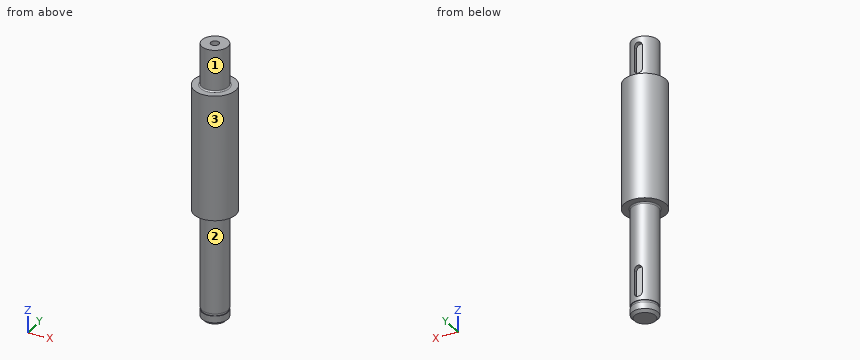
```python
from build123d import *

# Parameters (mm, degrees)
SKETCH1_R                          = 12.7
BOSS_EXTRUDE1_DEPTH                = 38.1
SKETCH3_R                          = 7.9375
BOSS_EXTRUDE2_DEPTH                = 66.675
SKETCH8_R                          = 12.7
SKETCH8_R_2                        = 7.4676
CUT_EXTRUDE1_DEPTH                 = 0.7112
BOSS_EXTRUDE3_START                = 25.4
SKETCH9_R                          = 7.9375
BOSS_EXTRUDE3_DEPTH                = 25.4
FILLET1_R                          = 0.79375
F_1_4_20_TAPPED_HOLE1_D            = 5.1054
F_1_4_20_TAPPED_HOLE1_DEPTH        = 38.1
F_1_4_20_TAPPED_HOLE1_TIP          = 1.533816902
F_3_16_START                       = 5.19049
F_3_16_0_1875_DIAMETER_SLOT1_DEPTH = 3.80951
CHAMFER1_SIZE                      = 1.5875


with BuildPart() as part:
    # Sketch1 → Boss-Extrude1 (new, symmetric)
    with BuildSketch(Plane.XY):
        with Locations(Location((0, 0, 0), (0, 0, 180))):
            Circle(SKETCH1_R)
    extrude(amount=BOSS_EXTRUDE1_DEPTH, both=True)

    # Sketch3 → Boss-Extrude2 (add)
    with BuildSketch(Plane(origin=(0, 0, -38.1), x_dir=(-1, 0, 0), z_dir=(0, 0, -1))):
        with Locations(Location((0, 0, 0), (0, 0, 180))):
            Circle(SKETCH3_R)
    extrude(amount=BOSS_EXTRUDE2_DEPTH)

    # Sketch8 → Cut-Extrude1 (cut, symmetric)
    with BuildSketch(Plane(origin=(0, 0, -98.425), x_dir=(-1, 0, 0), z_dir=(0, 0, -1))):
        Circle(SKETCH8_R)
        Circle(SKETCH8_R_2, mode=Mode.SUBTRACT)
    extrude(amount=CUT_EXTRUDE1_DEPTH, both=True, mode=Mode.SUBTRACT)

    # Sketch9 → Boss-Extrude3 (add)
    with BuildSketch(Plane.XY.offset(38.1).offset(BOSS_EXTRUDE3_START)):
        Circle(SKETCH9_R)
    extrude(amount=-BOSS_EXTRUDE3_DEPTH)

    # Fillet1
    fillet1_edges = [part.edges().sort_by_distance(p)[0] for p in [
        (-7.9375, 0, 38.1),
        (-7.9375, 0, -38.1),
    ]]
    fillet(fillet1_edges, radius=FILLET1_R)

    # 1/4-20 Tapped Hole1
    with Locations(Plane.XY.offset(63.5)):
        with Locations((0, 0)):
            Hole(F_1_4_20_TAPPED_HOLE1_D / 2, depth=F_1_4_20_TAPPED_HOLE1_DEPTH)
            with Locations((0, 0, -(F_1_4_20_TAPPED_HOLE1_DEPTH + F_1_4_20_TAPPED_HOLE1_TIP / 2))):  # 118° drill point
                Cone(0, F_1_4_20_TAPPED_HOLE1_D / 2, F_1_4_20_TAPPED_HOLE1_TIP, mode=Mode.SUBTRACT)

    # 3/16 (0.1875) Diameter Slot1: read off the stored shape, not the designer's step
    # 3/16 (0.1875) Diameter Slot1 outline → 3/16 (0.1875) Diameter Slot1 (cut)
    with BuildSketch(Plane(origin=(0, 0, 0), x_dir=(1, 0, 0), z_dir=(0, 1, 0)).offset(F_3_16_START)):
        with BuildLine():
            ThreePointArc((2.38125, -43.65625), (0, -41.275), (-2.38125, -43.65625))
            Line((-2.38125, -43.65625), (-2.38125, -57.94375))
            ThreePointArc((-2.38125, -57.94375), (0, -60.325), (2.38125, -57.94375))
            Line((2.38125, -57.94375), (2.38125, -43.65625))
        make_face()
        with BuildLine():
            ThreePointArc((2.38125, 92.86875), (0, 95.25), (-2.38125, 92.86875))
            Line((-2.38125, 92.86875), (-2.38125, 78.58125))
            ThreePointArc((-2.38125, 78.58125), (0, 76.2), (2.38125, 78.58125))
            Line((2.38125, 78.58125), (2.38125, 92.86875))
        make_face()
    extrude(amount=F_3_16_0_1875_DIAMETER_SLOT1_DEPTH, mode=Mode.SUBTRACT)

    # Chamfer1
    chamfer1_edges = [part.edges().sort_by_distance(p)[0] for p in [
        (-7.9375, 0, -104.775),
    ]]
    chamfer(chamfer1_edges, length=CHAMFER1_SIZE)


solid = part.part
```
CAD build for the part. Positions are in the model's coordinates, mm. Face numbers are marked on the shaded views. A direction names the side the tool comes from. Round coordinates to 2 decimals unless told otherwise and drop trailing zeros. Loops run counter-clockwise (first coordinate to the right, second up) from the corner with the lowest first, then second, coordinate; pieces in that order, holes last. Notation, with made-up numbers: M 52,31 L 102,31 A12 cw 102,39 Z; hole C 46,60 d4. An arc over 180 degrees is marked long. Use a Markdown table: item, result. Add a question column.
(1) Cut at B-B (z = 17.5). Give the cut face in (x, y), and give its area (3 significant figures).
(2) Cut at C-C (z = -62). Give the cut face in (x, y) (1 decimal).
(3) Flat gauge pins, fed straight in: pin 1 (4 mm diameter, centred on x = 0.5, z = 46.5, fed in from +Y); pin 2 (12 mm diameter, centred on y = 3, z = -75, fed in from -X); pin 3 (4 mm diameter, centred on y = -6, z = 26, fed in from -X). Where does each tip first touch, or does it go through?
(4) Which spindle directions (+Z, -Z, +X, -X, +Y, -Y) get a long thin tool onto all of the face, cutting with end or side? Do the marked faces 1, 2 and 3. Say none if no direction does.
(5) Cut at A-A (z = 48.5). Give the cut face in (x, y) (1 decimal).
(6) Drill centre lines: line 1 (Y direction, x = 0, z = 52); line 2 (Z direction, x = -8, y = 6.25); line 3 (Y direction, x = -0.75, z = 12.5). Where is each one in solid material? Low to high.
Geometry says:
| question | item | result |
|---|---|---|
| 1 | outline | C 0,0 d25.4 |
| 1 | area | 507 mm² |
| 2 | outline | C 0,0 d15.9 |
| 3 | pin 1 | stops at y = 7.57 |
| 3 | pin 2 | stops at x = -7.94 |
| 3 | pin 3 | stops at x = -12.05 |
| 4 | face 1 | +Z |
| 4 | face 2 | -Z |
| 4 | face 3 | +Z, -Z |
| 5 | outline | M -2.4,5.2 L -2.4,7.6 A7.9 ccw long 2.4,7.6 L 2.4,5.2 Z; hole C 0,0 d5.1 |
| 6 | line 1 | y = -7.94 to -2.55, 2.55 to 5.19 |
| 6 | line 2 | z = -38.1 to 38.1 |
| 6 | line 3 | y = -12.68 to 12.68 |
